Print and shaded views of the part. All mm, measured from the part's lowest x, y and z. Round coordinates to 2 decimals unless told otherwise and drop trailing zeros. Order: outer loops, then holes, each group sorted by start corner. A loop starts at its lowest first (then second) coordinate and runs counter-clockwise, first axis right, second up. Notation, with made-up numbers: M 75.25,12 L 80.25,12 A26 cw 80.25,47 Z; hole C 35,9 d5. An arc over 180 degrees is marked long. Write each question's results on one line, items separated by ' | '. Start each with the question number.
1. Band-saw the part on C-C, the plane z = 1.55. List the corners of the cut face in (x, y).
2. Band-saw the part on B-B, the plane x = 86.5. List the corners of the cut face in (y, z) (1 decimal).
3. Drop flat-ended pins along their axis: pin 1 Ø1.5 at (x, z) = (73.5, 2.5) entering from -Y; pin 2 Ø1.5 at (x, z) = (20.5, 3) entering from -Y; pin 3 Ø1.8 at (x, y) = (67.01, 72.5) entering from -Z; pin 4 Ø2 at (x, z) = (95.5, 1.5) entering from +Y (1 decimal). Give the stop position or say it passes through.
4. Band-saw the part on A-A, the plane y = 80. List the corners of the cut face in (x, z).
5. Band-saw the part on D-D, the plane y = 15.5. List the corners of the cut face in (x, z), then the cut area to 3 significant figures.
6. Probe L1, parallel to Y at x = 80, z = 2.2; L2, parallel to Y at x = 72, z = 2.4; L3, parallel to Y at x = 24.5, z = 1.4 (1 decimal). List the from-to ranges inside material, lowest first. Write a range as [from, to].
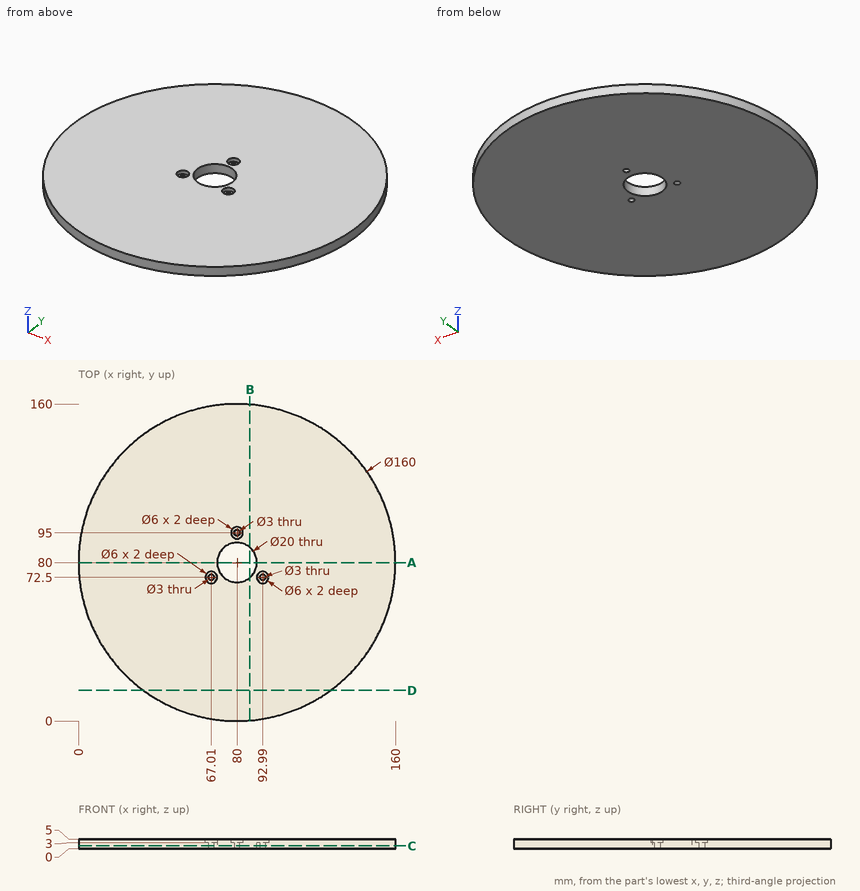
Solution:
1) outline: C 80,80 d160; hole C 67.01,72.5 d3; hole C 80,80 d20; hole C 80,95 d3; hole C 92.99,72.5 d3
2) outline: M 0.3,0 L 72.4,0 L 72.4,5 L 0.3,5 Z; M 87.6,0 L 159.7,0 L 159.7,5 L 87.6,5 Z
3) pin 1: y = 0.21 | pin 2: y = 25.7 | pin 3: through | pin 4: y = 158.7
4) outline: M 0,0 L 70,0 L 70,5 L 0,5 Z; M 90,0 L 160,0 L 160,5 L 90,5 Z
5) outline: M 32.67,0 L 127.33,0 L 127.33,5 L 32.67,5 Z | area: 473 mm^2
6) L1: [0, 70], [90, 93.5], [96.5, 160] | L2: [0.4, 74], [86, 159.6] | L3: [22.4, 137.6]
